Drawing for the job (mm, zero at the part's lowest x, y, z). Give positions to 0.01 mm unless a question says otherwise; leave off trailing zeros. Order: outer loops, then holes, each group sorted by start corner. A loop starts at its lowest first (then second) coordinate and runs counter-clockwise, first axis right, second up. Notation, with made-up numbers: (80, -31) - (131, -31) arc R13 cw to (131, -13) - close; hole circle Ø6 at (-17, 83.5). An arc over 180 degrees is marked (long way). Use a Markdown table: item, result. Add a question column.
(1) Wall check: line 1 (Y direction, x = 6.35, z = 0.6) (1 decimal); line 2 (Y direction, x = 17.5, z = 0.95); line 3 (Y direction, x = 26, z = 0.1). Give the ranges that are in metal, low to high.
(2) Slice it at A-A (x = 14). Write the cut outline in (y, z).
(3) Slice it at B-B (z = 0.95). Count the separate pieces of the cut face and the enclosed holes in it, then the cut area to 3 significant figures.
(4) Slice it at D-D (y = 6.35). Write the cut outline in (x, z) (1 decimal).
(5) Slice it at C-C (y = 57.15). Write the cut outline in (x, z) (1 decimal).
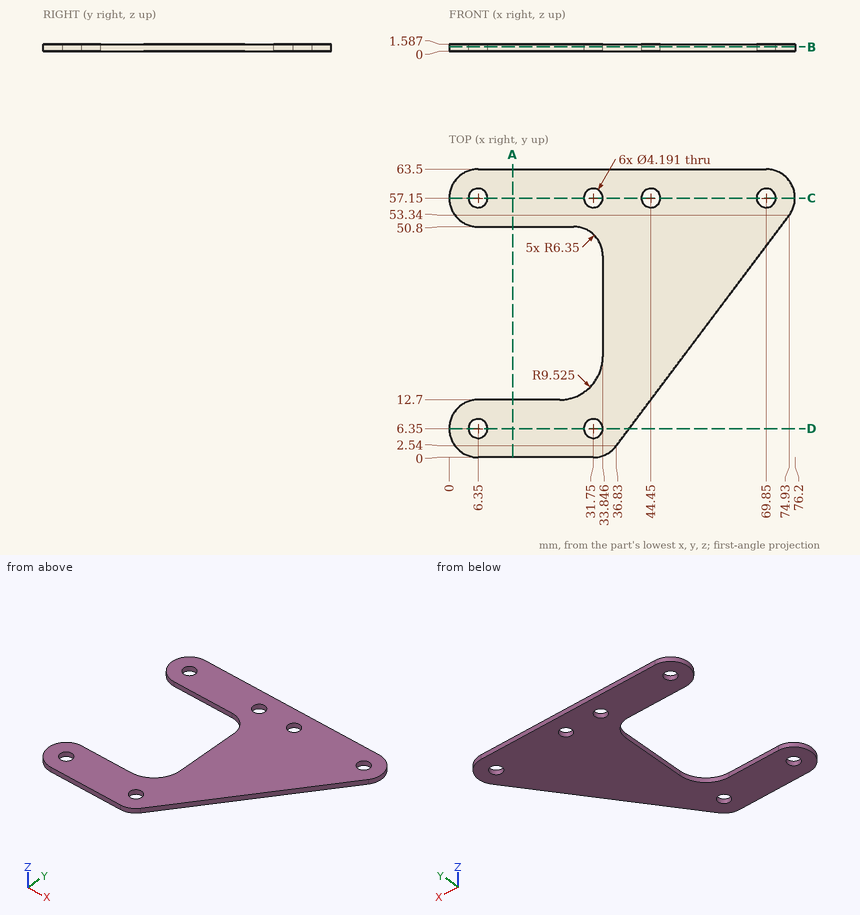
Solution:
| question | item | result |
|---|---|---|
| 1 | line 1 | 0 to 4.3, 8.4 to 12.7, 50.8 to 55.1, 59.2 to 63.5 |
| 1 | line 2 | 0 to 12.7, 50.8 to 63.5 |
| 1 | line 3 | 0 to 12.85, 50.8 to 63.5 |
| 2 | outline | (0, 0) - (12.7, 0) - (12.7, 1.59) - (0, 1.59) - close; (50.8, 0) - (63.5, 0) - (63.5, 1.59) - (50.8, 1.59) - close |
| 3 | separate pieces | 1 |
| 3 | enclosed holes | 6 |
| 3 | area | 2,310 mm2 |
| 4 | outline | (0, 0) - (4.3, 0) - (4.3, 1.6) - (0, 1.6) - close; (8.4, 0) - (29.7, 0) - (29.7, 1.6) - (8.4, 1.6) - close; (33.8, 0) - (39.7, 0) - (39.7, 1.6) - (33.8, 1.6) - close |
| 5 | outline | (0, 0) - (4.3, 0) - (4.3, 1.6) - (0, 1.6) - close; (8.4, 0) - (29.7, 0) - (29.7, 1.6) - (8.4, 1.6) - close; (33.8, 0) - (42.4, 0) - (42.4, 1.6) - (33.8, 1.6) - close; (46.5, 0) - (67.8, 0) - (67.8, 1.6) - (46.5, 1.6) - close; (71.9, 0) - (76.2, 0) - (76.2, 1.6) - (71.9, 1.6) - close |
